Here's how the part is built. I have some questions about the finished solid (model axes, mm). A direction names the side the tool comes from. Round coordinates to 2 decimals unless told otherwise and drop trailing zeros. Write each loop counter-clockwise with the first axis right and the second up, starting at its lowest first coordinate (ties: lowest second). Pieces come first, ordered by that corner, then holes. Notation, with made-up numbers: (69, -1) - (128, -1) arc R25 ccw to (128, 13) - close; hole circle Ø7 at (-38, 7). An arc over 180 degrees is marked (long way). Write item = value, one per line. Start each with the question number.
Item 1: Thinking about a two-plate mould opening in Z: for faces 4 (the face through (6, 2, 0)), 5 (the face through (12.38, -2.36, -0.12)), 6 (the face through (5.39, 3.15, -0.04)), 7 (the face through (8, -1, 2.4)), which applies, pulls with the +Z half, pulls with the -Z half, needs draft (parallel to the pull), parting line crosses it, or undercut?
Item 2: If I drill on line 1 along Z through (x, y) = (5.75, 0); line 2 along Z through (x, y) = (3.5, 0); line 3 along X through (y, z) = (2, -0.45), over which ranges is the centre line in solid material (lowest first)? Write a range as [from, to].
Item 3: Which directions (+Z, -Z, +X, -X, +Y, -Y) give clear straight access to the entire face, cutting with the end or side of a thin tool? Please do faces 1 (the face through (10, -0.5, -2)), 2 (the face through (2.22, -0.29, 2.23)), 3 (the face through (8.84, -3.15, 0.04)).
Item 4: If we section it at D-D (x = 12): Please give me the cut outline in (y, z).
Item 5: If we section it at A-A (z = 0): Please give me the cut outline in (x, y).
Item 6: For P1, Ø1, axis at x = 2.5, z = -0.5, coming from the -Y side; P2, Ø1.5, axis at x = 9.5, z = 1, coming from the -Y side, each with a flat end and sliding along its axis, tell me the tip position at first contact or that it passes through.
Item 7: If we section it at C-C (x = 3.5): Please give me the cut outline in (y, z), and give its area (3 significant figures).
Item 8: If we section it at B-B (y = 0): Please give me the cut outline in (x, z), and give its area (3 significant figures).
```python
from build123d import *

# Parameters (mm, degrees)
CUT_EXTRUDE_1_DEPTH      = 7
CHAMFER_1_SIZE           = 0.3
CHAMFER_1_SIZE2          = 0.824243226
SKETCH_3_R               = 0.4
CUT_EXTRUDE_2_DEPTH      = 10
CUT_EXTRUDE_3_DEPTH      = 7.0000001
CUT_EXTRUDE_3_DEPTH_BACK = 8.0000001


with BuildPart() as part:
    # Эскиз1 → Повернуть1 (revolve)
    with BuildSketch(Plane.XY):
        Polygon((0, 1.65), (13, 1.65), (13, 3.15), (4.5, 3.15), (4.5, 2.25), (0, 2.25), align=None)
    revolve(axis=Axis((0, 0, 0), (1, 0, 0)))

    # Эскиз2 → Вырез-Вытянуть1 (cut)
    with BuildSketch(Plane(origin=(13, 0, 0), x_dir=(0, 0, -1), z_dir=(1, 0, 0))):
        Polygon((-27.602946028, -0.5), (-3.110064308, -0.5), (3.110064308, -0.5), (27.602946028, -0.5), (27.602946028, 48.485763441), (-27.602946028, 48.485763441), align=None)
    extrude(amount=-CUT_EXTRUDE_1_DEPTH, mode=Mode.SUBTRACT)

    # Фаска1
    chamfer_1_edges = [part.edges().sort_by_distance(p)[0] for p in [
        (4.5, -3.15, 0),
    ]]
    chamfer_1_side = [part.faces().sort_by_distance(p)[0] for p in [
        (8.75, -3.15, 0),
    ]]
    chamfer(chamfer_1_edges, length=CHAMFER_1_SIZE, length2=CHAMFER_1_SIZE2, reference=chamfer_1_side[0])

    # Эскиз3 → Вырез-Вытянуть2 (cut)
    with BuildSketch(Plane(origin=(0, -0.5, 0), x_dir=(1, 0, 0), z_dir=(0, 1, 0))):
        with Locations((12, 0)):
            Circle(SKETCH_3_R)
    extrude(amount=-CUT_EXTRUDE_2_DEPTH, mode=Mode.SUBTRACT)

    # Эскиз4 → Вырез-Вытянуть3 (cut, two sides)
    with BuildSketch(Plane.ZY.offset(-6)) as cut_extrude_3_sk:
        with BuildLine():
            ThreePointArc((-3.110064308, -0.5), (-3.033707684, 0.84800807), (-2.4, 2.040220576))
            Line((-2.4, 2.040220576), (-3.699342341, 2.040220576))
            Line((-3.699342341, 2.040220576), (-3.699342341, -2.040220576))
            Line((-3.699342341, -2.040220576), (-2.4, -2.040220576))
            Line((-2.4, -2.040220576), (-2.4, -0.5))
            Line((-2.4, -0.5), (-3.110064308, -0.5))
        make_face()
        with BuildLine():
            Line((4.02795857, 2.040220576), (2.4, 2.040220576))
            ThreePointArc((2.4, 2.040220576), (3.033707684, 0.84800807), (3.110064308, -0.5))
            Line((3.110064308, -0.5), (2.4, -0.5))
            Line((2.4, -0.5), (2.4, -2.040220576))
            Line((2.4, -2.040220576), (4.02795857, -2.040220576))
            Line((4.02795857, -2.040220576), (4.02795857, 2.040220576))
        make_face()
        with BuildLine():
            Line((-2.4, -0.5), (-2.4, 2.040220576))
            ThreePointArc((-2.4, 2.040220576), (-3.033707684, 0.84800807), (-3.110064308, -0.5))
            Line((-3.110064308, -0.5), (-2.4, -0.5))
        make_face()
        with BuildLine():
            ThreePointArc((3.110064308, -0.5), (3.033707684, 0.84800807), (2.4, 2.040220576))
            Line((2.4, 2.040220576), (2.4, -0.5))
            Line((2.4, -0.5), (3.110064308, -0.5))
        make_face()
    extrude(amount=CUT_EXTRUDE_3_DEPTH, mode=Mode.SUBTRACT)
    extrude(cut_extrude_3_sk.sketch, amount=-CUT_EXTRUDE_3_DEPTH_BACK, mode=Mode.SUBTRACT)


solid = part.part
```
Reply:
q1.face_4 = needs draft
q1.face_5 = undercut
q1.face_6 = parting line crosses it
q1.face_7 = pulls with the +Z half
q2.line_1 = [-2.4, -1.65], [1.65, 2.4]
q2.line_2 = [-2.25, -1.65], [1.65, 2.25]
q2.line_3 = [0, 6]
q3.face_1 = +Z, -Z, +X, +Y
q3.face_2 = -X
q3.face_3 = +X, -X, -Y
q4.outline = (-3.12, -0.4) arc R3.15 ccw to (-2.04, -2.4) - (-0.5, -2.4) - (-0.5, -1.57) arc R1.65 cw to (-1.6, -0.4) - close; (-3.12, 0.4) - (-1.6, 0.4) arc R1.65 cw to (-0.5, 1.57) - (-0.5, 2.4) - (-2.04, 2.4) arc R3.15 ccw to start
q5.outline = (0, -2.25) - (4.5, -2.25) - (4.5, -2.33) - (4.8, -3.15) - (11.6, -3.15) - (11.6, -1.65) - (0, -1.65) - close; (0, 1.65) - (6, 1.65) - (6, 3.15) - (4.8, 3.15) - (4.5, 2.33) - (4.5, 2.25) - (0, 2.25) - close; (12.4, -3.15) - (13, -3.15) - (13, -1.65) - (12.4, -1.65) - close
q6.P1 = -2.25
q6.P2 = -3.14
q7.outline = circle Ø4.5 at (0, 0); hole circle Ø3.3 at (0, 0)
q7.area = 7.35 mm2
q8.outline = (0, -2.25) - (4.5, -2.25) - (4.5, -2.33) - (4.53, -2.4) - (6, -2.4) - (6, -1.65) - (0, -1.65) - close; (0, 1.65) - (6, 1.65) - (6, 2.4) - (4.53, 2.4) - (4.5, 2.33) - (4.5, 2.25) - (0, 2.25) - close
q8.area = 7.65 mm2
